from build123d import *

# Parameters (mm, degrees)
CHAMFER1_SIZE      = 0.25
CHAMFER2_SIZE      = 0.5
SKETCH2_R          = 4.275
CUT_EXTRUDE1_DEPTH = 1


with BuildPart() as part:
    # Sketch1 → Revolve1 (revolve)
    with BuildSketch(Plane(origin=(0, 0, 0), x_dir=(1, 0, 0), z_dir=(0, 1, 0))):
        Polygon((0, 0.35), (-3.75, 0.35), (-7.9, 2.746003617), (-10.15, 2.746003617), (-15, 6.815636828), (-15, 10.36), (-14.8, 10.36), (-14.8, 11.36), (-15, 11.36), (-15, 12.36), (-14.8, 12.36), (-14.8, 17.36), (-15.75, 17.36), (-15.75, 24.16), (-14, 24.16), (-14, 40.729872981), (-11.5, 45.06), (-9.16, 45.06), (-9.16, 46.06), (-10.16, 46.06), (-10.16, 48.96), (-9.16, 48.96), (-9.16, 49.96), (0, 49.96), align=None)
    revolve(axis=Axis((0, 0, -49.96), (0, 0, 1)))

    # Chamfer1
    # the kernel refuses this chamfer: 0.25 mm, written as the material it takes off along each edge
    with BuildSketch(Plane(origin=(0, 0, -12.36), x_dir=(-1, 0, 0), z_dir=(0, 1, 0))) as chamfer1_piece_1_section:
        Polygon((15, CHAMFER1_SIZE), (15 - CHAMFER1_SIZE, 0), (15, 0), align=None)
    chamfer1_piece_1 = revolve(axis=Axis((0, 0, -12.36), (0, 0, 1)), mode=Mode.PRIVATE)
    chamfer1_piece_1 = chamfer1_piece_1 - Plane(origin=(0, 0, -12.216726666), x_dir=(-1, 0, 0), z_dir=(0, 0, -1)) * Cylinder(14.8, 60, mode=Mode.PRIVATE)
    add(chamfer1_piece_1, mode=Mode.SUBTRACT)
    with BuildSketch(Plane(origin=(0, 0, -48.96), x_dir=(-1, 0, 0), z_dir=(0, 1, 0))) as chamfer1_piece_2:
        Polygon((10.16, CHAMFER1_SIZE), (10.16 - CHAMFER1_SIZE, 0), (10.16, 0), align=None)
    revolve(axis=Axis((0, 0, -48.96), (0, 0, 1)), mode=Mode.SUBTRACT)
    with BuildSketch(Plane(origin=(0, 0, -46.06), x_dir=(-1, 0, 0), z_dir=(0, 1, 0))) as chamfer1_piece_3:
        Polygon((10.16 - CHAMFER1_SIZE, 0), (10.16, -CHAMFER1_SIZE), (10.16, 0), align=None)
    revolve(axis=Axis((0, 0, -46.06), (0, 0, 1)), mode=Mode.SUBTRACT)

    # Chamfer2
    chamfer2_edges = [part.edges().sort_by_distance(p)[0] for p in [
        (15.75, 0, -24.16),
        (15.75, 0, -17.36),
    ]]
    chamfer(chamfer2_edges, length=CHAMFER2_SIZE)

    # Sketch2 → Cut-Extrude1 (cut)
    with BuildSketch(Plane(origin=(0, 0, -49.96), x_dir=(-1, 0, 0), z_dir=(0, 0, -1))):
        Circle(SKETCH2_R)
    extrude(amount=-CUT_EXTRUDE1_DEPTH, mode=Mode.SUBTRACT)


solid = part.part
Source: CAD feature listing. Evaluate the final solid. Frame: model axes, mm. A direction names the side the tool comes from. Coordinates: 2 decimals unless noted, no trailing zeros. Loops run counter-clockwise (first coordinate to the right, second up) from the corner with the lowest first, then second, coordinate; pieces in that order, holes last. Notation, with made-up numbers: (79.25, 88.25) -> (88.25, 88.25) arc R19 ccw to (88.25, 114.25) -> close; hole circle Ø2 at (58, 71.25). An arc over 180 degrees is marked (long way). Answer in a Markdown table with one row per item. Add a question column.
Q1. Section B-B on z = -19.5. Return the cut outline in (x, y), and give its area (3 significant figures).
Q2. Reachability of faces 1 (the face through (-1, -15, -17.36)), 2 (the face through (1.323, -10.074, -47.527)), 3 (the face through (-3.824, -1.204, -0.5)) from +Z, -Z, +X, -X, +Y, -Y: full face, straight path, thin tool, end or side. Return the list, or none.
Q3. Pull-direction query (Y, two-part tool) for faces 4 (the face through (0, 8.2, -2.746)), 5 (the face through (3.208, 14.448, -10.867)), 6 (the face through (0, 0, -48.96)); classes: pulls with the +Y half, pulls with the -Y half, needs draft (parallel to the pull), parting line crosses it, or undercut.
Q4. Contact query for flat-ended pins moving along their axis: pin 1 Ø8 at (y, z) = (-3.5, -38) entering from -X; pin 2 Ø12 at (x, z) = (8.5, -9.5) entering from +Y; pin 3 Ø12 at (x, y) = (12.5, 12) entering from -Z. Output: stop coordinate, or through.
Q5. Ray query, line 1 along Y through (x, z) = (0, -49.5) (3 decimals); line 2 along Z through (x, y) = (9.5, -11.5); line 3 along Z through (x, y) = (-4.5, 14.5). Return the intervals inside material, ascending.
Q6. Section A-A on z = -37. Return the cut outline in (x, y), and give its area (3 significant figures).
Computed values:
| question | item | result |
|---|---|---|
| 1 | outline | circle Ø31.5 at (0, 0) |
| 1 | area | 779 mm^2 |
| 2 | face 1 | none |
| 2 | face 2 | -Z |
| 2 | face 3 | +Z |
| 3 | face 4 | needs draft |
| 3 | face 5 | parting line crosses it |
| 3 | face 6 | undercut |
| 4 | pin 1 | stops at x = -14 |
| 4 | pin 2 | stops at y = 14.79 |
| 4 | pin 3 | stops at z = -45.06 |
| 5 | line 1 | y = -9.16 to -4.275, 4.275 to 9.16 |
| 5 | line 2 | z = -24.16 to -17.36, -12.19 to -11.36, -10.36 to -6.75 |
| 5 | line 3 | z = -24.16 to -17.36 |
| 6 | outline | circle Ø28 at (0, 0) |
| 6 | area | 616 mm^2 |
